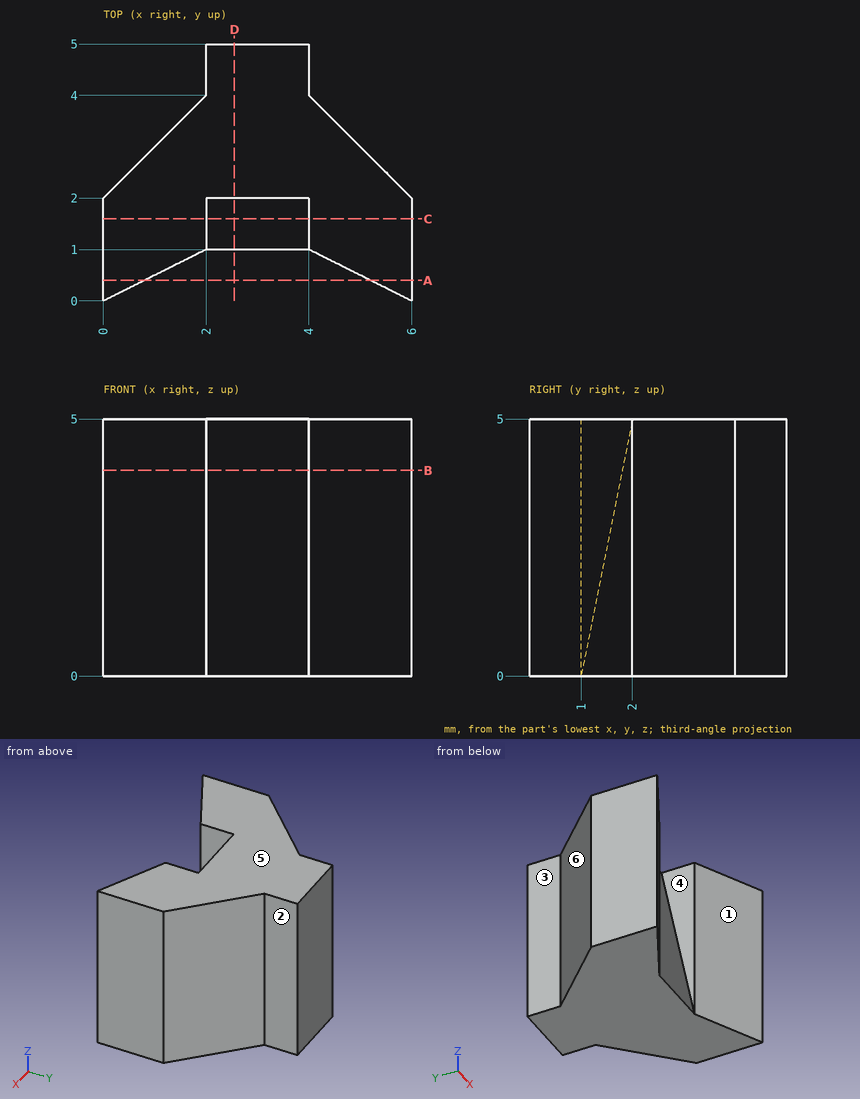
Part print with two shaded views. Sizes in mm from the minimum x, y, z corner. A direction names the side the tool comes from. Coordinates: 2 decimals unless noted, no trailing zeros. Write each loop counter-clockwise with the first axis right and the second up, starting at its lowest first coordinate (ties: lowest second). Pieces come first, ordered by that corner, then holes. Notation, with made-up numbers: (31.5, 57.25) - (37.5, 57.25) arc R11 cw to (37.5, 76.25) - close; hole circle Ø10 at (12.25, 40). An arc over 180 degrees is marked (long way). One line per item, written item: value. Start each with the question number.
1. Flat gauge pins, fed straight in: pin 1 (1.5 mm diameter, centred on x = 5, y = 4.5, fed in from +Z); pin 2 (0.5 mm diameter, centred on y = 4.5, z = 2, fed in from +X); pin 3 (0.5 mm diameter, centred on y = 4.5, z = 1.5, fed in from -X). Where does each tip first touch, or does it go through?
2. Slice it at A-A (y = 0.4). Write the cut outline in (x, z).
3. Slice it at D-D (x = 2.55). Write the cut outline in (y, z).
4. Mould opens along X. For the marked faces 4, 5 and 6 say: released by +X, released by -X, zero draft, split by the parting line, or undercut.
5. Slice it at C-C (y = 1.6). Write the cut outline in (x, z).
6. Tool access for the marked faces 1, 2 and 3: list every direction of +Z, -Z, +X, -X, +Y, -Y with a clear straight run to the whole face (end or side of a thin tool).
7. Probe line 1 (X direction, y = 1.4, z = 2.8); line 2 (X direction, y = 4.2, z = 3.75); line 3 (X direction, y = 0.35, z = 2.75). List the from-to ranges inside material, lowest first. Write a range as from..to.
8. Slice it at B-B (z = 4). Write the cut outline in (x, y).
Answers below:
1. pin 1: passes through
1. pin 2: stops at x = 4
1. pin 3: stops at x = 2
2. outline: (0, 0) - (0.8, 0) - (0.8, 5) - (0, 5) - close; (5.2, 0) - (6, 0) - (6, 5) - (5.2, 5) - close
3. outline: (1, 0) - (5, 0) - (5, 5) - (2, 5) - close
4. face 4: undercut
4. face 5: zero draft
4. face 6: released by -X
5. outline: (0, 0) - (6, 0) - (6, 5) - (4, 5) - (4, 3) - (2, 3) - (2, 5) - (0, 5) - close
6. face 1: +Z, -Z, -Y
6. face 2: +Z, -Z, +X, +Y
6. face 3: +Z, -Z, -X, +Y
7. line 1: x = 0..2, 4..6
7. line 2: x = 2..4
7. line 3: x = 0..0.7, 5.3..6
8. outline: (0, 0) - (2, 1) - (2, 1.8) - (4, 1.8) - (4, 1) - (6, 0) - (6, 2) - (4, 4) - (4, 5) - (2, 5) - (2, 4) - (0, 2) - close
